from build123d import *

# Parameters (mm, degrees)
ESQUISSE1_W                         = 85
ESQUISSE1_H                         = 10
ESQUISSE1_R                         = 1
BOSS_EXTRU_1_DEPTH                  = 3
ESQUISSE2_W                         = 165
ESQUISSE2_H                         = 65
BOSS_EXTRU_2_DEPTH                  = 3
ENL_V_MAT_EXTRU_1_REACH             = 87
ESQUISSE3_W                         = 34
ESQUISSE3_H                         = 35
ESQUISSE3_W_2                       = 71
BOSS_EXTRU_3_DEPTH                  = 10
BOSS_EXTRU_5_DEPTH                  = 30
ENL_V_MAT_EXTRU_2_REACH             = 87
ESQUISSE8_R                         = 1.65
ENL_V_MAT_EXTRU_2_DIRECTION_2_DEPTH = 1
ENL_V_MAT_EXTRU_3_DEPTH             = 8
ESQUISSE12_W                        = 95.226934881
ESQUISSE12_H                        = 85.849602385
ENL_V_MAT_EXTRU_4_DEPTH             = 66
ESQUISSE13_W                        = 60
ESQUISSE13_H                        = 20
BOSS_EXTRU_6_DEPTH                  = 3
ENL_V_MAT_EXTRU_5_DEPTH             = 3


with BuildPart() as part:
    # Esquisse1 → Boss.-Extru.1 (new body)
    with BuildSketch(Plane.XY):
        with Locations((42.5, 5)):
            Rectangle(ESQUISSE1_W, ESQUISSE1_H)
        with Locations((5, 5)):
            Circle(ESQUISSE1_R, mode=Mode.SUBTRACT)
    extrude(amount=BOSS_EXTRU_1_DEPTH)

    # Esquisse2 → Boss.-Extru.2 (add)
    with BuildSketch(Plane(origin=(85, 0, 0), x_dir=(0, 0, -1), z_dir=(1, 0, 0))):
        with Locations((17, -22.5)):
            Rectangle(ESQUISSE2_W, ESQUISSE2_H)
    extrude(amount=-BOSS_EXTRU_2_DEPTH)

    # Esquisse3 → Enlèv. mat.-Extru.1 (cut, up to next)
    with BuildSketch(Plane(origin=(85, 0, 0), x_dir=(0, 0, -1), z_dir=(1, 0, 0)), mode=Mode.PRIVATE) as enl_v_mat_extru_1_sk1:
        with Locations((-48.5, -7.5)):
            Rectangle(ESQUISSE3_W, ESQUISSE3_H)
    enl_v_mat_extru_1_tool1 = extrude(enl_v_mat_extru_1_sk1.sketch, amount=-ENL_V_MAT_EXTRU_1_REACH, mode=Mode.PRIVATE) & part.part
    add(enl_v_mat_extru_1_tool1.solids().sort_by_distance((85, -7.5, 48.5))[0], mode=Mode.SUBTRACT)
    # Esquisse3 → Enlèv. mat.-Extru.1 (cut, up to next)
    with BuildSketch(Plane(origin=(85, 0, 0), x_dir=(0, 0, -1), z_dir=(1, 0, 0)), mode=Mode.PRIVATE) as enl_v_mat_extru_1_sk2:
        with Locations((64, -7.5)):
            Rectangle(ESQUISSE3_W_2, ESQUISSE3_H)
    enl_v_mat_extru_1_tool2 = extrude(enl_v_mat_extru_1_sk2.sketch, amount=-ENL_V_MAT_EXTRU_1_REACH, mode=Mode.PRIVATE) & part.part
    add(enl_v_mat_extru_1_tool2.solids().sort_by_distance((85, -7.5, -64))[0], mode=Mode.SUBTRACT)

    # Esquisse5 → Boss.-Extru.3 (add)
    with BuildSketch(Plane(origin=(0, 10, 0), x_dir=(1, 0, 0), z_dir=(0, 1, 0))):
        Polygon((63.707714548, 0), (82, 28.5), (82, 0), align=None)
        Polygon((63.707714548, -3), (82, -3), (82, -31.5), align=None)
    extrude(amount=-BOSS_EXTRU_3_DEPTH)

    # Esquisse7 → Boss.-Extru.5 (add)
    with BuildSketch(Plane.XZ.offset(55)):
        Polygon((85, 65.5), (72.009618943, 73), (70.509618943, 70.401923789), (82, 63.767949192), align=None)
        Polygon((70.509618943, -104.401923789), (82, -97.767949192), (85, -99.5), (72.009618943, -107), align=None)
    extrude(amount=-BOSS_EXTRU_5_DEPTH)

    # Esquisse8 → Enlèv. mat.-Extru.2 (cut, up to next)
    with BuildSketch(Plane(origin=(85, 0, 0), x_dir=(0, 0, -1), z_dir=(1, 0, 0)), mode=Mode.PRIVATE) as enl_v_mat_extru_2_sk1:
        with Locations((-21.5, 5)):
            Circle(ESQUISSE8_R)
    enl_v_mat_extru_2_tool1 = extrude(enl_v_mat_extru_2_sk1.sketch, amount=-ENL_V_MAT_EXTRU_2_REACH, mode=Mode.PRIVATE) & part.part
    add(enl_v_mat_extru_2_tool1.solids().sort_by_distance((85, 5, 21.5))[0], mode=Mode.SUBTRACT)
    # Esquisse8 → Enlèv. mat.-Extru.2 (cut, up to next)
    with BuildSketch(Plane(origin=(85, 0, 0), x_dir=(0, 0, -1), z_dir=(1, 0, 0)), mode=Mode.PRIVATE) as enl_v_mat_extru_2_sk2:
        with Locations((18.5, 5)):
            Circle(ESQUISSE8_R)
    enl_v_mat_extru_2_tool2 = extrude(enl_v_mat_extru_2_sk2.sketch, amount=-ENL_V_MAT_EXTRU_2_REACH, mode=Mode.PRIVATE) & part.part
    add(enl_v_mat_extru_2_tool2.solids().sort_by_distance((85, 5, -18.5))[0], mode=Mode.SUBTRACT)

    # Esquisse8 → Enlèv. mat.-Extru.2 direction 2 (cut)
    with BuildSketch(Plane(origin=(85, 0, 0), x_dir=(0, 0, -1), z_dir=(1, 0, 0))):
        with Locations((-21.5, 5)):
            Circle(ESQUISSE8_R)
        with Locations((18.5, 5)):
            Circle(ESQUISSE8_R)
    extrude(amount=ENL_V_MAT_EXTRU_2_DIRECTION_2_DEPTH, mode=Mode.SUBTRACT)

    # Esquisse9 → Enlèv. mat.-Extru.3 (cut)
    with BuildSketch(Plane.ZY.offset(-72)):
        Polygon((-16.854551733, 7.85), (-20.145448267, 7.85), (-21.790896534, 5), (-20.145448267, 2.15), (-16.854551733, 2.15), (-15.209103466, 5), align=None)
        Polygon((23.145448267, 7.85), (19.854551733, 7.85), (18.209103466, 5), (19.854551733, 2.15), (23.145448267, 2.15), (24.790896534, 5), align=None)
    extrude(amount=-ENL_V_MAT_EXTRU_3_DEPTH, mode=Mode.SUBTRACT)

    # Esquisse12 → Enlèv. mat.-Extru.4 (cut, through all)
    with BuildSketch(Plane(origin=(0, 10, 0), x_dir=(1, 0, 0), z_dir=(0, 1, 0))):
        with Locations((34.386532559, 2.239892923)):
            Rectangle(ESQUISSE12_W, ESQUISSE12_H)
    extrude(amount=-ENL_V_MAT_EXTRU_4_DEPTH, mode=Mode.SUBTRACT)

    # Esquisse13 → Boss.-Extru.6 (add)
    with BuildSketch(Plane.ZY.offset(-82)):
        with Locations((1.5, 20)):
            Rectangle(ESQUISSE13_W, ESQUISSE13_H)
    extrude(amount=-BOSS_EXTRU_6_DEPTH)

    # Esquisse14 → Enlèv. mat.-Extru.5 (cut)
    with BuildSketch(Plane.ZY.offset(-82)):
        with BuildLine():
            Line((-20.15, -5), (-20.15, 25))
            ThreePointArc((-20.15, 25), (-18.5, 26.65), (-16.85, 25))
            Line((-16.85, 25), (-16.85, -5))
            ThreePointArc((-16.85, -5), (-18.5, -6.65), (-20.15, -5))
        make_face()
        with BuildLine():
            Line((19.85, -5), (19.85, 25))
            ThreePointArc((19.85, 25), (21.5, 26.65), (23.15, 25))
            Line((23.15, 25), (23.15, -5))
            ThreePointArc((23.15, -5), (21.5, -6.65), (19.85, -5))
        make_face()
    extrude(amount=-ENL_V_MAT_EXTRU_5_DEPTH, mode=Mode.SUBTRACT)


solid = part.part
Geometry check sheet. Reference: the model listing, model coordinates, mm. A direction names the side the tool comes from. Give positions to 0.01 mm unless a question says otherwise; leave off trailing zeros. Loops run counter-clockwise (first coordinate to the right, second up) from the corner with the lowest first, then second, coordinate; pieces in that order, holes last. Notation, with made-up numbers: (40.5, 46.5) -> (87.5, 46.5) arc R19 ccw to (87.5, 79.5) -> close; hole circle Ø3 at (7.25, 30). An arc over 180 degrees is marked (long way). Answer in a Markdown table with one row per item. Add a question column.
1) Cross-section at A-A on y = -3. Record the boundary of the cut face in (x, z), and give its area (3 significant figures).
2) Cross-section at C-C on x = 79.5. Record the boundary of the cut face in (y, z), and give its area (3 significant figures).
3) Gauge pin test, flat ends, axial feed: P1, Ø3.5, axis at x = 83.5, y = 17, coming from the +Z side; P2, Ø1.5, axis at x = 83, y = 9, coming from the -Z side; P3, Ø12, axis at y = -13, z = 25.5, coming from the -X side. Record the tip position at first contact, or that the pin passes through.
4) Cross-section at D-D on y = -38. Record the boundary of the cut face in (x, z), and give its area (3 significant figures).
5) Cross-section at B-B on z = 21.5. Record the boundary of the cut face in (x, y).
6) Draft check along Y on faces 5 (the face through (83, 10, 23.15)), 6 (the face through (83, 30, 1)), 7 (the face through (83, 10, -20.15)), 8 (the face through (76.174, -40.21, -101.131)). Enter one of: pulls with the +Y half, pulls with the -Y half, needs draft (parallel to the pull), parting line crosses it, or undercut.
7) Material ranges on probe 1 along X at (y, z) = (-30, 2); probe 2 along Z at (x, y) = (78, -42.5); probe 3 along Y at (x, z) = (83.75, 66), recorded low to high. Write a range as from..to.
8) Set-up check for faces 1 (the face through (83, 2, 31.5)), 2 (the face through (82, -31, -18)), 3 (the face through (83.48, 26.65, -18.54)), 4 (the face through (83, -25, -70)): record each of +Z, -Z, +X, -X, +Y, -Y from which the full face is reachable in a straight line by a thin tool's end or side.
Outcome:
| question | item | result |
|---|---|---|
| 1 | outline | (82, -28.5) -> (85, -28.5) -> (85, -20.15) -> (82, -20.15) -> close; (82, -16.85) -> (85, -16.85) -> (85, 19.85) -> (82, 19.85) -> close; (82, 23.15) -> (85, 23.15) -> (85, 31.5) -> (82, 31.5) -> close |
| 1 | area | 160 mm^2 |
| 2 | outline | (-55, -102.68) -> (-25, -102.68) -> (-25, -99.21) -> (-55, -99.21) -> close; (-55, 65.21) -> (-25, 65.21) -> (-25, 68.68) -> (-55, 68.68) -> close |
| 2 | area | 208 mm^2 |
| 3 | P1 | stops at z = 31.5 |
| 3 | P2 | stops at z = -28.5 |
| 3 | P3 | stops at x = 82 |
| 4 | outline | (70.51, -104.4) -> (72.01, -107) -> (85, -99.5) -> (85, 65.5) -> (72.01, 73) -> (70.51, 70.4) -> (82, 63.77) -> (82, -97.77) -> close |
| 4 | area | 575 mm^2 |
| 5 | outline | (82, -55) -> (85, -55) -> (85, -6.65) -> (82, -6.65) -> close; (82, 26.65) -> (85, 26.65) -> (85, 30) -> (82, 30) -> close |
| 6 | face 5 | undercut |
| 6 | face 6 | pulls with the +Y half |
| 6 | face 7 | undercut |
| 6 | face 8 | needs draft |
| 7 | probe 1 | x = 82..85 |
| 7 | probe 2 | z = -103.54..-100.08, 66.08..69.54 |
| 7 | probe 3 | y = -55..-25 |
| 8 | face 1 | +Z, +X, -X, +Y |
| 8 | face 2 | -X, +Y, -Y |
| 8 | face 3 | +X, -X |
| 8 | face 4 | -Z, +X, -X, +Y |
